Input: part model. Units: mm. Frame: model coordinates. Coordinates: 2 decimals unless noted, no trailing zeros. Write each loop counter-clockwise with the first axis right and the second up, starting at its lowest first coordinate (ties: lowest second). Pieces come first, ordered by that corner, then holes. Notation, with made-up numbers: M -8.5,77.5 L 9.5,77.5 A27 ccw 9.5,97.5 Z; hole C -11.75,-34.5 d11. An arc over 180 degrees is marked long. Write each question's results on one line, items separated by ' | '. Start each with the question number.
1. Section query C-C, the plane z = 15. Output: boundary loops of the cut face in (x, y), and give its area (3 significant figures).
2. Pull-direction query (X, two-part tool) for faces 1 (the cylindrical face through (-42.1, 2.6, 55.2)), 2 (the cylindrical face through (1.4, 2.58, -10.26)), 3 (the flat face through (0, 3, -35.56)), 4 (the cylindrical face through (0.3, 2.5, -22.8)); classes: +X half, -X half, draft (parallel to the pull), parting line (faces both ways), or undercut.
3. Ray query, probe 1 along X at (y, z) = (1.2, 21.59); probe 2 along X at (y, z) = (2.65, -20.32); probe 3 along X at (y, z) = (1.65, 44.45). Return the intervals inside material, ascending.
4. Section query B-B, the plane y = 3.3. Output: boundary loops of the cut face in (x, z).
5. Section query A-A, the plane x = 0. Output: boundary loops of the cut face in (y, z), and give its area (3 significant figures).
6. First-contact query: pin 1 (3 mm diameter, centred on x = -34.5, z = 25.5, fed in from -Y). Flat tip, straight axial feed; report the tip coordinate or a pass-through.
7. Section query D-D, the plane x = 33.02. Output: boundary loops of the cut face in (y, z).
```python
from build123d import *

# Parameters (mm, degrees)
SKETCH2_W                 = 95
SKETCH2_H                 = 96.52
BOSS_EXTRUDE3_DEPTH       = 5.08
SKETCH3_R                 = 31.879999994
CUT_EXTRUDE1_DEPTH        = 78.447905072
M6X1_0_TAPPED_HOLE1_D     = 5
M6X1_0_TAPPED_HOLE1_DEPTH = 5.08
M6X1_0_TAPPED_HOLE1_TIP   = 1.502151548
SKETCH7_R                 = 2.54
CUT_EXTRUDE2_DEPTH        = 7.62
FILLET1_R                 = 19.05


with BuildPart() as part:
    # Sketch2 → Boss-Extrude3 (new body)
    with BuildSketch(Plane(origin=(0, 0, 0), x_dir=(1, 0, 0), z_dir=(0, 1, 0))):
        with Locations((0, -12.7)):
            Rectangle(SKETCH2_W, SKETCH2_H)
    extrude(amount=BOSS_EXTRUDE3_DEPTH)

    # Sketch3 → Cut-Extrude1 (cut, through all)
    with BuildSketch(Plane(origin=(0, 5.08, 0), x_dir=(1, 0, 0), z_dir=(0, 1, 0))):
        with Locations(Location((0, -21.59, 0), (0, 0, 270))):
            Circle(SKETCH3_R)
    extrude(amount=-CUT_EXTRUDE1_DEPTH, mode=Mode.SUBTRACT)

    # M6x1.0 Tapped Hole1
    with Locations(Plane(origin=(0, 5.08, 0), x_dir=(1, 0, 0), z_dir=(0, 1, 0))):
        with Locations((-40, 20.32), (40, 20.32), (0, 20.32)):
            Hole(M6X1_0_TAPPED_HOLE1_D / 2, depth=M6X1_0_TAPPED_HOLE1_DEPTH)
            with Locations((0, 0, -(M6X1_0_TAPPED_HOLE1_DEPTH + M6X1_0_TAPPED_HOLE1_TIP / 2))):  # 118° drill point
                Cone(0, M6X1_0_TAPPED_HOLE1_D / 2, M6X1_0_TAPPED_HOLE1_TIP, mode=Mode.SUBTRACT)

    # Sketch7 → Cut-Extrude2 (cut)
    with BuildSketch(Plane(origin=(0, 5.08, 0), x_dir=(1, 0, 0), z_dir=(0, 1, 0))):
        with Locations(Location((-33.02, -44.45, 0), (0, 0, 270))):
            Circle(SKETCH7_R)
        with Locations(Location((33.02, -44.45, 0), (0, 0, 270))):
            Circle(SKETCH7_R)
    extrude(amount=-CUT_EXTRUDE2_DEPTH, mode=Mode.SUBTRACT)

    # Fillet1
    fillet1_edges = [part.edges().sort_by_distance(p)[0] for p in [
        (47.5, 2.54, -35.56),
        (47.5, 2.54, 60.96),
        (-47.5, 2.54, 60.96),
        (-47.5, 2.54, -35.56),
    ]]
    fillet(fillet1_edges, radius=FILLET1_R)


solid = part.part
```
Answer:
1) outline: M -47.5,0 L -31.19,0 L -31.19,5.08 L -47.5,5.08 Z; M 31.19,0 L 47.5,0 L 47.5,5.08 L 31.19,5.08 Z | area: 166 mm^2
2) face 1: -X half | face 2: undercut | face 3: draft | face 4: undercut
3) probe 1: -47.5 to -31.88, 31.88 to 47.5 | probe 2: -47.12 to -42.5, -37.5 to -2.5, 2.5 to 37.5, 42.5 to 47.12 | probe 3: -47.33 to -35.56, -30.48 to -22.22, 22.22 to 30.48, 35.56 to 47.33
4) outline: M -47.5,-16.51 A19.05 ccw -28.45,-35.56 L 28.45,-35.56 A19.05 ccw 47.5,-16.51 L 47.5,41.91 A19.05 ccw 28.45,60.96 L -28.45,60.96 A19.05 ccw -47.5,41.91 Z; hole C -40,-20.32 d5; hole C -33.02,44.45 d5.08; hole C 0,21.59 d63.76; hole C 0,-20.32 d5; hole C 33.02,44.45 d5.08; hole C 40,-20.32 d5
5) outline: M 0,-35.56 L 5.08,-35.56 L 5.08,-22.82 L 0,-22.82 Z; M 0,-17.82 L 5.08,-17.82 L 5.08,-10.29 L 0,-10.29 Z; M 0,53.47 L 5.08,53.47 L 5.08,60.96 L 0,60.96 Z | area: 141 mm^2
6) pin 1: y = 0
7) outline: M 0,-35 L 5.08,-35 L 5.08,41.91 L 0,41.91 Z; M 0,46.99 L 5.08,46.99 L 5.08,60.4 L 0,60.4 Z
